Geometry check sheet. Reference: the model listing, model coordinates, mm. A direction names the side the tool comes from. Give positions to 0.01 mm unless a question says otherwise; leave off trailing zeros. Order: outer loops, then holes, each group sorted by start corner. A loop starts at its lowest first (then second) coordinate and runs counter-clockwise, first axis right, second up. Notation, with made-up numbers: M -38.5,-39 L 1.5,-39 A11 cw 1.5,-26 Z; hole C 32,-17.5 d2. An arc over 180 degrees is marked long. Answer as CSV lines item,"result". Start each with the question number.
Q1. Set-up check for faces 4 (the flat face through (3, 53.975, 2)), 5 (the flat face through (60.325, 56, 2)), 6 (the flat face through (93.218, 9, 2)), 7 (the flat face through (-2, 15.875, 2)): record each of +Z, -Z, +X, -X, +Y, -Y from which the full face is reachable in a straight line by a thin tool's end or side.
Q2. Section check D-D, the plane x = 6. Record the boundary of the cut face in (y, z) (3 decimals).
Q3. Thickness scan on line 1 (X direction, y = 30, z = 1.8); line 2 (X direction, y = 6.5, z = 0.5); line 3 (Y direction, x = 31.75, z = 0.7) (3 decimals). Record the ranges inside material, lowest first.
Q4. Section check B-B, the plane x = 31.75. Record the boundary of the cut face in (y, z) (3 decimals), then the cut area to 3 significant figures.
Q5. Section check A-A, the plane y = 6.35. Record the boundary of the cut face in (x, z) (3 decimals).
Q6. Go/stop test with flat-tipped pins: pin 1 (4 mm diameter, centred on x = 61.47, y = 30.15, fed in from +Z); pin 2 (1 mm diameter, centred on x = -1, z = 2, fed in from -Y) (3 decimals); pin 3 (1.6 mm diameter, centred on y = 55, z = 2, fed in from -X) (3 decimals); pin 4 (8 mm diameter, centred on x = 87.5, y = 44, fed in from -Z). Record where each tip stops, or that it passes through.
Q7. Section check C-C, the plane z = 0.7. Record the boundary of the cut face in (x, y) (3 decimals).
Q8. Mould release check, pull along Y, two halves, no side actions. Record for faces 1 (the cylindrical face through (31.2, 27.67, 1.57)), 2 (the flat face through (101, 24.075, 2)), 3 (the flat face through (47.625, 56, 2)): +Y half, -Y half, draft (parallel to the pull), parting line (faces both ways), or undercut.
```python
from build123d import *

# Parameters (mm, degrees)
SKETCH1_R           = 2.54
BOSS_EXTRUDE1_DEPTH = 3.175
FILLET1_R           = 6.35


with BuildPart() as part:
    # Sketch1 → Boss-Extrude1 (new body)
    with BuildSketch(Plane.XY):
        Polygon((0, 15.875), (0, 0), (93.218, 0), (93.218, 24.07511214), (101.6, 24.07511214), (101.6, 57.15), (60.325, 57.15), (60.325, 53.975), (47.625, 53.975), (47.625, 57.15), (34.925, 57.15), (34.925, 53.975), (22.225, 53.975), (22.225, 57.15), (9.525, 57.15), (9.525, 53.975), (-3.175, 53.975), (-3.175, 41.275), (0, 41.275), (0, 28.575), (-3.175, 28.575), (-3.175, 15.875), align=None)
        with Locations((40.259, 6.35)):
            Circle(SKETCH1_R, mode=Mode.SUBTRACT)
        with Locations((52.959, 6.35)):
            Circle(SKETCH1_R, mode=Mode.SUBTRACT)
        with Locations((31.75, 30.1498)):
            Circle(SKETCH1_R, mode=Mode.SUBTRACT)
        with Locations((61.468, 30.1498)):
            Circle(SKETCH1_R, mode=Mode.SUBTRACT)
        with Locations((91.186, 30.1498)):
            Circle(SKETCH1_R, mode=Mode.SUBTRACT)
    extrude(amount=BOSS_EXTRUDE1_DEPTH)

    # Fillet1
    fillet1_edges = [part.edges().sort_by_distance(p)[0] for p in [
        (93.218, 24.07511214, 1.5875),
    ]]
    fillet(fillet1_edges, radius=FILLET1_R)


solid = part.part
```
Answer block:
1,face 4,"+Z, -Z, -X, +Y"
1,face 5,"+Z, -Z, +Y"
1,face 6,"+Z, -Z, +X, -Y"
1,face 7,"+Z, -Z, -X, -Y"
2,outline,"M 0,0 L 53.975,0 L 53.975,3.175 L 0,3.175 Z"
3,line 1,"x = 0 to 29.21, 34.29 to 58.93, 64 to 88.65, 93.72 to 101.6"
3,line 2,"x = 0 to 37.72, 42.79 to 50.42, 55.49 to 93.22"
3,line 3,"y = 0 to 27.61, 32.69 to 53.975"
4,outline,"M 0,0 L 27.61,0 L 27.61,3.175 L 0,3.175 Z; M 32.69,0 L 53.975,0 L 53.975,3.175 L 32.69,3.175 Z"
4,area,"155 mm2"
5,outline,"M 0,0 L 37.719,0 L 37.719,3.175 L 0,3.175 Z; M 42.799,0 L 50.419,0 L 50.419,3.175 L 42.799,3.175 Z; M 55.499,0 L 93.218,0 L 93.218,3.175 L 55.499,3.175 Z"
6,pin 1,"passes through"
6,pin 2,"stops at y = 15.875"
6,pin 3,"stops at x = 9.525"
6,pin 4,"stops at z = 0"
7,outline,"M -3.175,15.875 L 0,15.875 L 0,0 L 93.218,0 L 93.218,17.725 A6.35 cw 99.568,24.075 L 101.6,24.075 L 101.6,57.15 L 60.325,57.15 L 60.325,53.975 L 47.625,53.975 L 47.625,57.15 L 34.925,57.15 L 34.925,53.975 L 22.225,53.975 L 22.225,57.15 L 9.525,57.15 L 9.525,53.975 L -3.175,53.975 L -3.175,41.275 L 0,41.275 L 0,28.575 L -3.175,28.575 Z; hole C 31.75,30.15 d5.08; hole C 40.259,6.35 d5.08; hole C 52.959,6.35 d5.08; hole C 61.468,30.15 d5.08; hole C 91.186,30.15 d5.08"
8,face 1,"undercut"
8,face 2,"-Y half"
8,face 3,"draft"
